CAD build for the part. Positions are in the model's coordinates, mm. A direction names the side the tool comes from. Give positions to 0.01 mm unless a question says otherwise; leave off trailing zeros. Loops run counter-clockwise (first coordinate to the right, second up) from the corner with the lowest first, then second, coordinate; pieces in that order, holes last. Notation, with made-up numbers: (-31, 29) -> (-27, 29) arc R30 cw to (-27, 57) -> close; hole circle Ø4 at (89, 79.25). An arc over 180 degrees is marked (long way). Use one line per item in the form item = value.
Autodesk Inventor part; units mm, degrees
ref_plane "Work Plane2" through (104.775, 0, 0) normal (1, 0, 0) x (0, 1, 0)
ref_plane "XZ Plane" through (0, 0, 0) normal (0, 1, 0) x (-1, 0, 0)
ref_plane "XY Plane" through (0, 0, 0) normal (0, 0, 1) x (1, 0, 0)
sketch "Sketch1" plane through (0, 0, 0) normal (0, 1, 0) x (-1, 0, 0)
  circle A0 centre (0, 0) radius 104.775
  dimension "baseOutsideDiameter" = 209.55
extrude "Extrusion1" add sketch "Sketch1" along normal blind 6.35
sketch "Sketch7" plane through (0, 6.35, 0) normal (0, 1, 0) x (1, 0, 0)
  line L0 (0, 0) -> (0, 104.775) construction
  circle A0 centre (0, 0) radius 104.775 construction
  line L1 (88.9, -55.449) -> (88.9, 55.449)
  arc A1 (88.9, -55.449) -> (88.9, 55.449) centre (0, 0) ccw
  dimension "spaceforTube" = 88.9
extrude "Extrusion7" add sketch "Sketch7" along normal blind 177.8
mirror "Mirror1" about plane through (0, 0, 0) normal (1, 0, 0) of "Extrusion7"
ref_plane "Work Plane2" through (104.775, 0, 0) normal (1, 0, 0) x (0, 1, 0)
sketch "Sketch8" plane through (104.775, 0, 0) normal (1, 0, 0) x (0, 1, 0)
  circle A0 centre (158.75, 0) radius 6.35
  line L0 (6.35, 55.449) -> (6.35, 104.775)
  point P0 (0, 0)
  dimension "d34" = 12.7
  dimension "holeHeight" = 152.4
extrude "Extrusion8" cut sketch "Sketch8" against normal through all
sketch "Sketch9" plane through (0, 0, 0) normal (0, -1, 0) x (1, 0, 0)
  circle A0 centre (0, 0) radius 6.35
  dimension "d47" = 12.7
extrude "Extrusion9" cut sketch "Sketch9" against normal through all
sketch "Sketch10" plane through (0, 0, 0) normal (0, -1, 0) x (1, 0, 0)
  point P0 (0, 0)
  point P1 (-50.8, 0)
  dimension "d50" = 50.8
hole "Hole1" at (-50.8, 0, 0) direction (0, 1, 0) diameter 6.7564 end through all
pattern_circular "Circular Pattern2" count 6 over 360 about axis through (0, -10, 0) along (0, 1, 0) of "Hole1"
equation "\"spaceforTube\" = bracketWidth + 0.5 * tubeDiameter"
equation "\"tubeDiameter\" = 165.1"
equation "\"bracketWidth\" = 6.35"
properties part number "topOfRaBase" material "ABS Plastic"
1. Tool access for faces 1 (the flat face through (-88.9, 94, -1)), 2 (the flat face through (-95, 184.15, -1)): list every direction of +Z, -Z, +X, -X, +Y, -Y with a clear straight run to the whole face (end or side of a thin tool).
Result sheet:
face_1 = +Z, -Z, +Y
face_2 = +Z, -Z, +X, -X, +Y
2. Drop flat-ended pins along their axis: P1, Ø2, axis at y = 109.5, z = -40, coming from the +X side; P2, Ø6, axis at x = 8, z = -81.5, coming from the +Y side; P3, Ø10, axis at x = 0, z = 0, coming from the -Y side; P4, Ø1, axis at y = 94, z = -46.5, coming from the +X side. Give the stop position or say it passes through.
Result sheet:
P1 = 97.25
P2 = 6.35
P3 = through
P4 = 94.14
3. Cut at D-D, the plane z = 32. Write the cut outline in (x, y), then the cut area to 3 significant figures.
Result sheet:
outline = (-99.77, 0) -> (99.77, 0) -> (99.77, 184.15) -> (88.9, 184.15) -> (88.9, 6.35) -> (-88.9, 6.35) -> (-88.9, 184.15) -> (-99.77, 184.15) -> close
area = 5,130 mm^2
4. Mould opens along Z. For faces 3 (the cylindrical face through (-28.698, 3.219, 43.262)), 4 (the flat face through (88.9, 94, 1)) say: pulls with the +Z half, pulls with the -Z half, needs draft (parallel to the pull), parting line crosses it, or undercut.
Result sheet:
face_3 = undercut
face_4 = needs draft
5. Drill centre lines: line 1 (Y direction, x = -95, z = 0); line 2 (Y direction, x = -53, z = -25.5); line 3 (X direction, y = 174.5, z = 3). Where is each one in solid material? Low to high.
Result sheet:
line_1 = 0 to 152.4, 165.1 to 184.15
line_2 = 0 to 6.35
line_3 = -104.73 to -88.9, 88.9 to 104.73
6. Cut at B-B, the plane y = 158.75. Write the cut outline in (x, z) (3 decimals), then the cut area to 3 significant figures.
Result sheet:
outline = (-104.582, -6.35) arc R104.775 ccw to (-88.9, -55.449) -> (-88.9, -6.35) -> close; (-104.582, 6.35) -> (-88.9, 6.35) -> (-88.9, 55.449) arc R104.775 ccw to start; (88.9, -55.449) arc R104.775 ccw to (104.582, -6.35) -> (88.9, -6.35) -> close; (88.9, 6.35) -> (104.582, 6.35) arc R104.775 ccw to (88.9, 55.449) -> close
area = 1,980 mm^2
7. Cut at A-A, the plane x = 0. Write the cut outline in (y, z) (3 decimals).
Result sheet:
outline = (0, -104.775) -> (6.35, -104.775) -> (6.35, -6.35) -> (0, -6.35) -> close; (0, 6.35) -> (6.35, 6.35) -> (6.35, 104.775) -> (0, 104.775) -> close
8. Cut at C-C, the plane y = 69. Write the cut outline in (x, z) (3 decimals).
Result sheet:
outline = (-88.9, -55.449) -> (-88.9, 55.449) arc R104.775 ccw to start; (88.9, -55.449) arc R104.775 ccw to (88.9, 55.449) -> close
